from build123d import *

# Parameters (mm, degrees)
F0_R     = 4.1
F1_DEPTH = 6.3
F0_R_2   = 6.5
F2_DEPTH = 3
F0_R_3   = 12.5
F3_DEPTH = 1.5
F4_R     = 0.5


# Not quite as in the source:
# - a fillet or chamfer that OpenCascade refuses, or shapes differently, is made with other operations: its cross-section is extruded or revolved along the edge and cut away or added
# - a feature names something its author has since deleted; it is built from what else it names


with BuildPart() as f1:
    # F0 (on Top) → F1 (new body)
    with BuildSketch(Plane.XY):
        Circle(F0_R)
    extrude(amount=F1_DEPTH)

    # F0 (on Top) → F2 (join)
    with BuildSketch(Plane.XY):
        Circle(F0_R_2)
        Circle(F0_R, mode=Mode.SUBTRACT)
    extrude(amount=F2_DEPTH)

    # F0 (on Top) → F3 (join)
    with BuildSketch(Plane.XY):
        Circle(F0_R_3)
        Circle(F0_R_2, mode=Mode.SUBTRACT)
    extrude(amount=F3_DEPTH)

    # F4
    f4_edges = [f1.edges().sort_by_distance(p)[0] for p in [
        (-4.1, 0, 6.3),
    ]]
    fillet(f4_edges, radius=F4_R)

    # F5: fillet of radius 2 on 1 edges, made by hand

    # F5_s1 → F5_t2 (revolve, cut)
    with BuildSketch(Plane.XZ):
        with BuildLine():
            ThreePointArc((12.5, 1.5), (11.7882531983, 0.4188611699), (10.5635083269, 0))
            Line((10.5635083269, 0), (12.5, 0))
            Line((12.5, 0), (12.5, 1.5))
        make_face()
    revolve(axis=Axis((0, 0, 0), (0, 0, 1)), mode=Mode.SUBTRACT)


solid = f1.part
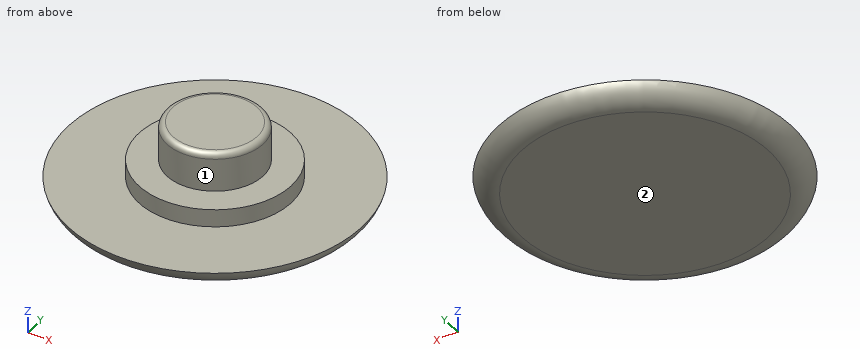
CAD build for the part. Positions are in the model's coordinates, mm. Face numbers are marked on the shaded views. A direction names the side the tool comes from. Round coordinates to 2 decimals unless told otherwise and drop trailing zeros. Write each loop counter-clockwise with the first axis right and the second up, starting at its lowest first coordinate (ties: lowest second). Pieces come first, ordered by that corner, then holes. Notation, with made-up numbers: M 71,15.5 L 111,15.5 A30 ccw 111,37.5 Z; hole C 39.25,69 d8. An arc over 180 degrees is marked long. Put each result on its own line as item: value. Start each with the question number.
1) Saw through at C-C, the plane z = 5. Write the cut outline in (x, y).
2) Pin check, flat tips, straight feed: pin 1 Ø1 at (x, y) = (6.5, -6) entering from +Z; pin 2 Ø6 at (x, y) = (3.5, -6) entering from +Z; pin 3 Ø10.5 at (x, y) = (2.5, 3) entering from +Z; pin 4 Ø1.5 at (x, z) = (4.5, 3.5) entering from +Y. Stop position of each tip, or through.
3) Drill centre lines: probe 1 along Z at (x, y) = (-9.25, 5); probe 2 along Z at (x, y) = (-5.25, 3); probe 3 along Y at (x, z) = (2.5, 5.5). Where is each one in solid material? Low to high. Write a range as [from, to].
4) 3-axis set-ups, long thin cutter, end or side, ignore diameter. For the marked faces 1 and 2: which of +Z, -Z, +X, -X, +Y, -Y reach the whole face in a straight line?
5) Saw through at A-A, the plane x = 0. Write the cut outline in (y, z).
Resolved:
1. outline: C 0,0 d8.2
2. pin 1: z = 1.5
2. pin 2: z = 6.16
2. pin 3: z = 6.3
2. pin 4: y = 5.17
3. probe 1: [0, 1.5]
3. probe 2: [0, 3]
3. probe 3: [-3.25, 3.25]
4. face 1: +Z
4. face 2: -Z, +X, -X, +Y, -Y
5. outline: M -12.5,1.5 A2 ccw -10.56,0 L 10.56,0 A2 ccw 12.5,1.5 L 6.5,1.5 L 6.5,3 L 4.1,3 L 4.1,5.8 A0.5 ccw 3.6,6.3 L -3.6,6.3 A0.5 ccw -4.1,5.8 L -4.1,3 L -6.5,3 L -6.5,1.5 Z
